Autodesk Inventor part; units mm, degrees
ref_plane "YZ Plane" through (0, 0, 0) normal (1, 0, 0) x (0, 1, 0)
ref_plane "XZ Plane" through (0, 0, 0) normal (0, 1, 0) x (-1, 0, 0)
ref_plane "XY Plane" through (0, 0, 0) normal (0, 0, 1) x (1, 0, 0)
sketch "Sketch1" plane through (0, 0, 0) normal (0, 0, 1) x (1, 0, 0)
  line L0 (0, 25.4) -> (-28.702, 25.4) construction
  line L1 (0, 25.4) -> (-93.98, 25.4) construction
  line L2 (-93.98, 25.4) -> (-90.805, 25.4) construction
  line L3 (-90.805, 25.4) -> (-84.455, 22.4389) construction
  line L4 (-90.805, 25.4) -> (-90.805, 22.4389) construction
  line L5 (-90.805, 0) -> (-93.98, 0)
  line L6 (-28.702, 59.6457) -> (-28.702, -91.9304) construction
  arc A0 (-28.9184, -9.248) -> (-32.3684, -1.8494) centre (-35.052, -7.6045) ccw
  line L7 (-74.93, -180.9657) -> (-28.702, -8.4405)
  line L8 (-90.805, 25.4) -> (-90.805, 0)
  line L9 (-90.805, 25.4) -> (-32.3684, -1.8494)
  line L10 (-28.702, -7.6045) -> (-60.452, -7.6045) construction
  line L11 (-60.452, 11.2462) -> (-60.452, -126.9331) construction
  line L12 (-60.452, -126.9331) -> (-54.102, -126.9331) construction
  line L13 (-54.102, -126.9331) -> (-54.102, -103.2346) construction
  line L14 (-54.102, -103.2346) -> (-60.452, -103.2346)
  line L15 (-60.452, 11.2462) -> (-60.452, 1.7212) construction
  line L16 (-60.452, 11.2462) -> (-60.452, 4.7154) construction
  line L17 (-60.452, 4.7154) -> (-46.4468, 4.7154)
  line L18 (-60.452, 4.7154) -> (-60.452, -103.2346)
  line L19 (-93.98, 0) -> (-93.98, -12.7) construction
  line L20 (-60.452, -12.7) -> (-73.152, -12.7) construction
  line L21 (-93.98, -12.7) -> (-93.98, -25.4) construction
  line L22 (-93.98, -25.4) -> (-93.98, -88.9) construction
  line L23 (-93.98, -88.9) -> (-81.28, -88.9) construction
  line L24 (-81.28, -88.9) -> (-81.28, -25.4) construction
  line L25 (-93.98, -25.4) -> (-81.28, -25.4)
  line L26 (-81.28, -25.4) -> (-81.28, -88.9)
  line L27 (-81.28, -88.9) -> (-93.98, -88.9)
  line L28 (-93.98, -12.7) -> (-73.152, -12.7)
  line L29 (-73.152, -138.7824) -> (-63.627, -138.7824)
  line L30 (-81.28, -88.9) -> (-81.28, -180.9657)
  line L31 (-81.28, -180.9657) -> (-74.93, -180.9657)
  line L32 (-73.152, -12.7) -> (-73.152, -138.7824)
  line L33 (-87.63, -25.4) -> (-87.63, -31.3436)
  line L34 (-87.63, -31.3436) -> (-93.98, -31.3436)
  line L35 (-93.98, 0) -> (-93.98, -25.4)
  line L36 (-93.98, -31.3436) -> (-93.98, -88.9)
  line L37 (-87.63, -155.5657) -> (-87.63, -216.5135)
  line L38 (-28.9184, -9.248) -> (-84.455, -216.5135)
  line L39 (-84.455, -216.5135) -> (-87.63, -216.5135)
  line L40 (-81.28, -155.5657) -> (-87.63, -155.5657)
  line L41 (-60.452, 4.7154) -> (-60.452, -7.6045)
  line L42 (-66.802, -38.1) -> (-73.152, -38.1)
  line L43 (-66.802, -38.1) -> (-66.802, 4.7154)
  line L44 (-66.802, 4.7154) -> (-60.452, 4.7154)
  line L45 (0, -319.0244) -> (0, 122.7573)
  point P0 (0, 0)
  point P1 (-93.98, -255.9127)
  point P2 (-88.7095, 22.4389)
  dimension "d0" = 28.702
  dimension "d1" = 93.98
  dimension "d2" = 3.175
  dimension "d3" = 25
  dimension "d5" = 25.4
  dimension "d6" = 25.4
  dimension "d8" = 12.7
  dimension "d12" = 31.75
  dimension "d13" = 6.35
  dimension "d16" = 12.7
  dimension "d17" = 12.7
  dimension "d18" = 12.7
  dimension "d19" = 63.5
  dimension "d20" = 12.7
  dimension "d22" = 9.525
  dimension "d23" = 6.35
  dimension "d25" = 5.9436
  dimension "d26" = 15
  dimension "d27" = 3.175
  dimension "d28" = 6.35
  dimension "d29" = 25.4
  dimension "d30" = 107.95
  dimension "d31" = 6.35
  dimension "d32" = 25.4
revolve "Revolution1" add sketch "Sketch1" angle 360 about axis through (0, -10, 0) along (0, 1, 0) contours L8 L9 L17 L44 L43 L42 L32 L28 L35 L5
properties part number "Phenolic" material "Phenolic Resin"
Build history of the part. All positions in model axes, mm. A direction names the side the tool comes from. Coordinates: 2 decimals unless noted, no trailing zeros. Order: outer loops, then holes, each group sorted by start corner. A loop starts at its lowest first (then second) coordinate and runs counter-clockwise, first axis right, second up. Notation, with made-up numbers: (-6, 57) -> (31, 57) arc R19 ccw to (31, 79) -> close; hole circle Ø11 at (52.5, 9.25). An arc over 180 degrees is marked (long way). Answer in a Markdown table with one row per item. Add a question column.
Q1. Which spindle directions (+Z, -Z, +X, -X, +Y, -Y) get a long thin tool onto all of the face, cutting with end or side? Do faces 4 (the face through (49, 0, 77)), 5 (the face through (20.373, -6.439, 91.745)), 6 (the face through (14.481, -16.393, -65.213)). Say none if no direction does.
Q2. Band-saw the part on A-A, the plane z = 0. List the corners of the cut face in (x, y) (3 decimals), then the cut area to 3 significant figures.
Q3. Band-saw the part on D-D, the plane y = -33. List the corners of the cut face in (x, z), then the cut area to 3 significant figures.
Q4. Drop flat-ended pins along their axis: pin 1 (10 mm diameter, centred on y = 1, z = 63, fed in from -X); pin 2 (1 mm diameter, centred on y = 18.5, z = 62, fed in from -X); pin 3 (3 mm diameter, centred on x = -43, y = -4.5, fed in from +Z). Give the stop position or say it passes through.
Q5. Mould opens along X. For faces 1 (the face through (-32, -38.1, -59)), 2 (the face through (-86.61, 12.52, -27.28)), 3 (the face through (-14, 4.715, 45)) say: +X half, -X half, draft (parallel to the pull), parting line (faces both ways), or undercut.
Q6. Wall check: line 1 along Z through (x, y) = (0, -8); line 2 along Z through (x, y) = (0, -24); line 3 along Y through (x, z) = (75, 51). Give the ranges that are in metal, low to high. Write a range as [from, to].
Q7. Band-saw the part on C-C, the plane y = 14. List the corners of the cut face in (x, z) (3 decimals).
Q8. Band-saw the part on B-B, the plane x = 0. List the corners of the cut face in (y, z) (3 decimals), then the cut area to 3 significant figures.
Answers follow:
| question | item | result |
|---|---|---|
| 1 | face 4 | +Y |
| 1 | face 5 | +Y, -Y |
| 1 | face 6 | -Y |
| 2 | outline | (-93.98, -12.7) -> (-73.152, -12.7) -> (-73.152, -38.1) -> (-66.802, -38.1) -> (-66.802, 4.715) -> (-46.447, 4.715) -> (-90.805, 25.4) -> (-90.805, 0) -> (-93.98, 0) -> close; (46.447, 4.715) -> (66.802, 4.715) -> (66.802, -38.1) -> (73.152, -38.1) -> (73.152, -12.7) -> (93.98, -12.7) -> (93.98, 0) -> (90.805, 0) -> (90.805, 25.4) -> close |
| 2 | area | 2,160 mm^2 |
| 3 | outline | circle Ø146.3 at (0, 0); hole circle Ø133.6 at (0, 0) |
| 3 | area | 2,790 mm^2 |
| 4 | pin 1 | x = -73.87 |
| 4 | pin 2 | x = -66.81 |
| 4 | pin 3 | z = 84.32 |
| 5 | face 1 | draft |
| 5 | face 2 | parting line |
| 5 | face 3 | undercut |
| 6 | line 1 | [-93.98, -66.8], [66.8, 93.98] |
| 6 | line 2 | [-73.15, -66.8], [66.8, 73.15] |
| 6 | line 3 | [-12.7, 25.35] |
| 7 | outline | circle Ø181.61 at (0, 0); hole circle Ø132.715 at (0, 0) |
| 8 | outline | (-38.1, -73.152) -> (-12.7, -73.152) -> (-12.7, -93.98) -> (0, -93.98) -> (0, -90.805) -> (25.4, -90.805) -> (4.715, -46.447) -> (4.715, -66.802) -> (-38.1, -66.802) -> close; (-38.1, 66.802) -> (4.715, 66.802) -> (4.715, 46.447) -> (25.4, 90.805) -> (0, 90.805) -> (0, 93.98) -> (-12.7, 93.98) -> (-12.7, 73.152) -> (-38.1, 73.152) -> close |
| 8 | area | 2,160 mm^2 |
